from build123d import *

# Parameters (mm, degrees)
SKETCH_W        = 80.5
SKETCH_H        = 40.5
PAD_DEPTH       = 8.6
POCKET_DEPTH    = 40.501
POCKET001_DEPTH = 80.501
SKETCH003_R     = 0.255
PAD001_DEPTH    = 6


with BuildPart() as part:
    # Sketch → Pad (new body)
    with BuildSketch(Plane.XY):
        with Locations((40.25, 20.25)):
            Rectangle(SKETCH_W, SKETCH_H)
    extrude(amount=PAD_DEPTH)

    # Sketch001 (on Face1 of Pad) → Pocket (cut, through all)
    with BuildSketch(Plane.XZ):
        Polygon((2, 0), (3, 1), (77.5, 1), (78.5, 0), align=None)
    extrude(amount=-POCKET_DEPTH, mode=Mode.SUBTRACT)

    # Sketch002 (on Face9 of Pocket) → Pocket001 (cut, through all)
    with BuildSketch(Plane(origin=(0, 0, 0), x_dir=(0, -1, 0), z_dir=(-1, 0, 0))):
        Polygon((-38.5, 0), (-37.5, 1), (-3, 1), (-2, 0), align=None)
    extrude(amount=-POCKET001_DEPTH, mode=Mode.SUBTRACT)

    # Sketch003 (on Face11 of Pocket001) → Pad001 (join)
    with BuildSketch(Plane(origin=(0, 0, 1), x_dir=(1, 0, 0), z_dir=(0, 0, -1))):
        with Locations((21.2, -5.12)):
            Circle(SKETCH003_R)
        with Locations((59.3, -5.12)):
            Circle(SKETCH003_R)
        with Locations((23.74, -5.12)):
            Circle(SKETCH003_R)
        with Locations((26.28, -5.12)):
            Circle(SKETCH003_R)
        with Locations((28.82, -5.12)):
            Circle(SKETCH003_R)
        with Locations((31.36, -5.12)):
            Circle(SKETCH003_R)
        with Locations((33.9, -5.12)):
            Circle(SKETCH003_R)
        with Locations((36.44, -5.12)):
            Circle(SKETCH003_R)
        with Locations((38.98, -5.12)):
            Circle(SKETCH003_R)
        with Locations((41.52, -5.12)):
            Circle(SKETCH003_R)
        with Locations((44.06, -5.12)):
            Circle(SKETCH003_R)
        with Locations((46.6, -5.12)):
            Circle(SKETCH003_R)
        with Locations((49.14, -5.12)):
            Circle(SKETCH003_R)
        with Locations((51.68, -5.12)):
            Circle(SKETCH003_R)
        with Locations((54.22, -5.12)):
            Circle(SKETCH003_R)
        with Locations((56.76, -5.12)):
            Circle(SKETCH003_R)
    pad001 = extrude(amount=PAD001_DEPTH)

    # Mirrored: Pad001 across Sketch003 Axis17
    add(pad001.mirror(Plane(origin=(0, 20.25, 1), x_dir=(0, 0, -1), z_dir=(0, -1, 0))))


solid = part.part
Geometry check sheet. Reference: the model listing, model coordinates, mm. Round coordinates to 2 decimals unless told otherwise and drop trailing zeros. Write each loop counter-clockwise with the first axis right and the second up, starting at its lowest first coordinate (ties: lowest second). Pieces come first, ordered by that corner, then holes.
Item 1: Material ranges on line 1 along Z through (x, y) = (40.5, 33), recorded low to high.
Determined:
line 1: z = 1 to 8.6
Item 2: Section check A-A (z = -3.25). Give the number of separate pieces and of enclosed holes in the cut face, plus the area to 3 significant figures.
Determined:
separate pieces: 32
enclosed holes: 0
area: 6.54 mm2
Item 3: Go/stop test with flat-tipped pins: pin 1 Ø1 at (x, y) = (80, 39) entering from -Z; pin 2 Ø1 at (x, z) = (33.5, -2.5) entering from +Y (3 decimals); pin 3 Ø4 at (x, y) = (19, 7) entering from -Z. Record where each tip stops, or that it passes through.
Determined:
pin 1: stops at z = 0
pin 2: stops at y = 35.635
pin 3: stops at z = 1
Item 4: Section check B-B (x = 61.5). Record the boundary of the cut face in (y, z).
Determined:
outline: (0, 1) - (40.5, 1) - (40.5, 8.6) - (0, 8.6) - close
Item 5: Section check C-C (y = 14). Record the boundary of the cut face in (x, z), plus the area to 3 significant figures.
Determined:
outline: (0, 1) - (80.5, 1) - (80.5, 8.6) - (0, 8.6) - close
area: 612 mm2
Item 6: Mould release check, pull along X, two halves, no side actions. Record for faces 1 (the face through (80.5, 20, 4)), 2 (the face through (0, 20, 4)), 3 (the face through (1, 40, 0)), 4 (the face through (40, 21, 1)): +X half, -X half, draft (parallel to the pull), parting line (faces both ways), or undercut.
Determined:
face 1: +X half
face 2: -X half
face 3: draft
face 4: undercut
